```python
from build123d import *

# Parameters (mm, degrees)
SZKIC1_R                    = 24
SZKIC1_R_2                  = 2.25
SZKIC1_R_3                  = 14
DODANIE_WYCI_GNI_CIE1_DEPTH = 5
SZKIC2_R                    = 5
SZKIC2_R_2                  = 22.5
DODANIE_WYCI_GNI_CIE2_DEPTH = 5


with BuildPart() as part:
    # Szkic1 → Dodanie-wyciągnięcie1 (new body)
    with BuildSketch(Plane.XY):
        Circle(SZKIC1_R)
        with Locations((0, 17.5)):
            Circle(SZKIC1_R_2, mode=Mode.SUBTRACT)
        with Locations((17.5, 0)):
            Circle(SZKIC1_R_2, mode=Mode.SUBTRACT)
        with Locations((0, -17.5)):
            Circle(SZKIC1_R_2, mode=Mode.SUBTRACT)
        with Locations((-17.5, 0)):
            Circle(SZKIC1_R_2, mode=Mode.SUBTRACT)
        Circle(SZKIC1_R_3, mode=Mode.SUBTRACT)
    extrude(amount=DODANIE_WYCI_GNI_CIE1_DEPTH)

    # Szkic2 → Dodanie-wyciągnięcie2 (add)
    with BuildSketch(Plane.XY.offset(5)):
        with BuildLine():
            ThreePointArc((10, 35), (0, 45), (-10, 35))
            ThreePointArc((-10, 35), (-17.32233047, 17.32233047), (-35, 10))
            ThreePointArc((-35, 10), (-45, 0), (-35, -10))
            ThreePointArc((-35, -10), (-17.32233047, -17.32233047), (-10, -35))
            ThreePointArc((-10, -35), (0, -45), (10, -35))
            ThreePointArc((10, -35), (17.32233047, -17.32233047), (35, -10))
            ThreePointArc((35, -10), (45, 0), (35, 10))
            ThreePointArc((35, 10), (17.32233047, 17.32233047), (10, 35))
        make_face()
        with Locations((0, -35)):
            Circle(SZKIC2_R, mode=Mode.SUBTRACT)
        with Locations((-35, 0)):
            Circle(SZKIC2_R, mode=Mode.SUBTRACT)
        Circle(SZKIC2_R_2, mode=Mode.SUBTRACT)
        with Locations((35, 0)):
            Circle(SZKIC2_R, mode=Mode.SUBTRACT)
        with Locations((0, 35)):
            Circle(SZKIC2_R, mode=Mode.SUBTRACT)
    extrude(amount=-DODANIE_WYCI_GNI_CIE2_DEPTH)


solid = part.part
```
Here's how the part is built. I have some questions about the finished solid (model axes, mm). Give positions to 0.01 mm unless a question says otherwise; leave off trailing zeros. Write each loop counter-clockwise with the first axis right and the second up, starting at its lowest first coordinate (ties: lowest second). Pieces come first, ordered by that corner, then holes. Notation, with made-up numbers: (-24, 83) -> (-10, 83) arc R20 ccw to (-10, 105) -> close; hole circle Ø7 at (-38.5, 55). An arc over 180 degrees is marked (long way). Write each question's results on one line, items separated by ' | '.
Item 1: Suppose I cut it at A-A on z = 1.2. Give the number of separate pieces and of enclosed holes in the cut face, plus the area to 3 significant figures.
Output:
separate pieces: 1 | enclosed holes: 9 | area: 2,570 mm^2
Item 2: Suppose I cut it at D-D on x = 32. Write out the boundary of the cut face in (y, z).
Output:
outline: (-10.18, 0) -> (-4, 0) -> (-4, 5) -> (-10.18, 5) -> close; (4, 0) -> (10.18, 0) -> (10.18, 5) -> (4, 5) -> close
Item 3: For pin 1 Ø2 at (x, z) = (19, 4.5) entering from +Y; pin 2 Ø2.5 at (x, y) = (0, 17.5) entering from -Z; pin 3 Ø2 at (x, z) = (16.5, 3.5) entering from -Y; pin 4 Ø1.5 at (y, z) = (7, 2) entering from -X, each with a flat end and sliding along its axis, tell me the tip position at first contact or that it passes through.
Output:
pin 1: stops at y = 16.67 | pin 2: passes through | pin 3: stops at y = -19.36 | pin 4: stops at x = -42.81
Item 4: If I drill on L1, parallel to Y at x = 0, z = 3.2; L2, parallel to X at y = 35.5, z = 3.25; L3, parallel to Y at x = 35, z = 4.1, over which ranges is the centre line in solid material (lowest first)?
Output:
L1: y = -45 to -40, -30 to -19.75, -15.25 to -14, 14 to 15.25, 19.75 to 30, 40 to 45 | L2: x = -9.99 to -4.97, 4.97 to 9.99 | L3: y = -10 to -5, 5 to 10
Item 5: Suppose I cut it at B-B on y = 0. Write out the boundary of the cut face in (x, z), plus the area to 3 significant figures.
Output:
outline: (-45, 0) -> (-40, 0) -> (-40, 5) -> (-45, 5) -> close; (-30, 0) -> (-19.75, 0) -> (-19.75, 5) -> (-30, 5) -> close; (-15.25, 0) -> (-14, 0) -> (-14, 5) -> (-15.25, 5) -> close; (14, 0) -> (15.25, 0) -> (15.25, 5) -> (14, 5) -> close; (19.75, 0) -> (30, 0) -> (30, 5) -> (19.75, 5) -> close; (40, 0) -> (45, 0) -> (45, 5) -> (40, 5) -> close | area: 165 mm^2
Item 6: We'd pull the mould along X, two halves only. Please class faces 1 (the face through (17.129, -17.518, 2.535)), 2 (the face through (6, 14, 0)), 3 (the face through (-0.488, 15.304, 2.465)): pulls with the +X half, pulls with the -X half, needs draft (parallel to the pull), parting line crosses it, or undercut.
Output:
face 1: pulls with the +X half | face 2: needs draft | face 3: undercut
